```python
from build123d import *

# Parameters (mm, degrees)
SKETCH1_W           = 88.9
SKETCH1_H           = 50.8
BOSS_EXTRUDE1_DEPTH = 6
SKETCH2_W           = 50.8
SKETCH2_H           = 19.05
BOSS_EXTRUDE2_DEPTH = 3
SKETCH3_R           = 1.5875
CUT_EXTRUDE1_DEPTH  = 97.234466279
SKETCH4_R           = 2
CUT_EXTRUDE2_DEPTH  = 58.092600221


with BuildPart() as part:
    # Sketch1 → Boss-Extrude1 (new body)
    with BuildSketch(Plane(origin=(0, 0, 0), x_dir=(1, 0, 0), z_dir=(0, 1, 0))):
        Rectangle(SKETCH1_W, SKETCH1_H)
    extrude(amount=BOSS_EXTRUDE1_DEPTH)

    # Sketch2 → Boss-Extrude2 (add)
    with BuildSketch(Plane.ZY.offset(44.45)):
        with Locations((0, -3.525)):
            Rectangle(SKETCH2_W, SKETCH2_H)
    boss_extrude2 = extrude(amount=BOSS_EXTRUDE2_DEPTH)

    # Sketch3 → Cut-Extrude1 (cut, through all)
    with BuildSketch(Plane.ZY.offset(47.45)):
        with Locations((-12.7, -9.875)):
            Circle(SKETCH3_R)
        with Locations((12.7, -9.875)):
            Circle(SKETCH3_R)
    cut_extrude1 = extrude(amount=-CUT_EXTRUDE1_DEPTH, mode=Mode.SUBTRACT)

    # Mirror1: Boss-Extrude2, Cut-Extrude1 across plane
    add(boss_extrude2.mirror(Plane(origin=(0, 0, 0), x_dir=(0, 0, 1), z_dir=(1, 0, 0))))
    add(cut_extrude1.mirror(Plane(origin=(0, 0, 0), x_dir=(0, 0, 1), z_dir=(1, 0, 0))), mode=Mode.SUBTRACT)

    # Sketch4 → Cut-Extrude2 (cut, through all)
    with BuildSketch(Plane(origin=(0, 6, 0), x_dir=(1, 0, 0), z_dir=(0, 1, 0))):
        with Locations(Location((-12.7, 12.7, 0), (0, 0, 270))):
            Circle(SKETCH4_R)
        with Locations(Location((12.7, 12.7, 0), (0, 0, 270))):
            Circle(SKETCH4_R)
        with Locations(Location((-12.7, -12.7, 0), (0, 0, 270))):
            Circle(SKETCH4_R)
        with Locations(Location((12.7, -12.7, 0), (0, 0, 270))):
            Circle(SKETCH4_R)
    extrude(amount=-CUT_EXTRUDE2_DEPTH, mode=Mode.SUBTRACT)


solid = part.part
```
Geometry check sheet. Reference: the model listing, model coordinates, mm. A direction names the side the tool comes from. Give positions to 0.01 mm unless a question says otherwise; leave off trailing zeros. Write each loop counter-clockwise with the first axis right and the second up, starting at its lowest first coordinate (ties: lowest second). Pieces come first, ordered by that corner, then holes.
1) Section check A-A, the plane z = -12.7. Record the boundary of the cut face in (x, y).
2) Section check C-C, the plane x = -35. Record the boundary of the cut face in (y, z), and give its area (3 significant figures).
3) Access from +Z, -Z, +X, -X, +Y, -Y to the whole of each face (thin tool, end or side, straight path). Record for faces 1 (the flat face through (-44.45, -6, 0)), 2 (the flat face through (0, 2, -25.4)).
4) Section check B-B, the plane x = -12.7. Record the boundary of the cut face in (y, z), and give its area (3 significant figures).
5) Release check for a two-part mould opening along X. For faces 3 (the cylindrical face through (-45.971, -9.398, -11.186)), 4 (the flat face through (47.45, -3, 0)), 5 (the cylindrical face through (11.934, 3.042, -10.853)) record: pulls with the +X half, pulls with the -X half, needs draft (parallel to the pull), parting line crosses it, or undercut.
6) Material ranges on L1, parallel to X at y = -6.5, z = -1; L2, parallel to X at y = 1.7, z = 12.7; L3, parallel to Y at x = -21, z = 14, recorded low to high.
7) Gauge pin test, flat ends, axial feed: pin 1 (12 mm diameter, centred on x = 15, z = 1.5, fed in from -Y); pin 2 (5 mm diameter, centred on y = -9.875, z = 12.7, fed in from -X). Record the tip position at first contact, or that the pin passes through.
Computed:
1. outline: (-47.45, -13.05) - (-44.45, -13.05) - (-44.45, -11.46) - (-47.45, -11.46) - close; (-47.45, -8.29) - (-44.45, -8.29) - (-44.45, 0) - (-14.7, 0) - (-14.7, 6) - (-47.45, 6) - close; (-10.7, 0) - (10.7, 0) - (10.7, 6) - (-10.7, 6) - close; (14.7, 0) - (44.45, 0) - (44.45, -8.29) - (47.45, -8.29) - (47.45, 6) - (14.7, 6) - close; (44.45, -13.05) - (47.45, -13.05) - (47.45, -11.46) - (44.45, -11.46) - close
2. outline: (0, -25.4) - (6, -25.4) - (6, 25.4) - (0, 25.4) - close
2. area: 305 mm2
3. face 1: +Z, -Z, -Y
3. face 2: -Z, +X, -X, +Y, -Y
4. outline: (0, -25.4) - (6, -25.4) - (6, -14.7) - (0, -14.7) - close; (0, -10.7) - (6, -10.7) - (6, 10.7) - (0, 10.7) - close; (0, 14.7) - (6, 14.7) - (6, 25.4) - (0, 25.4) - close
4. area: 257 mm2
5. face 3: needs draft
5. face 4: pulls with the +X half
5. face 5: undercut
6. L1: x = -47.45 to -44.45, 44.45 to 47.45
6. L2: x = -47.45 to -14.7, -10.7 to 10.7, 14.7 to 47.45
6. L3: y = 0 to 6
7. pin 1: stops at y = 0
7. pin 2: stops at x = -47.45
